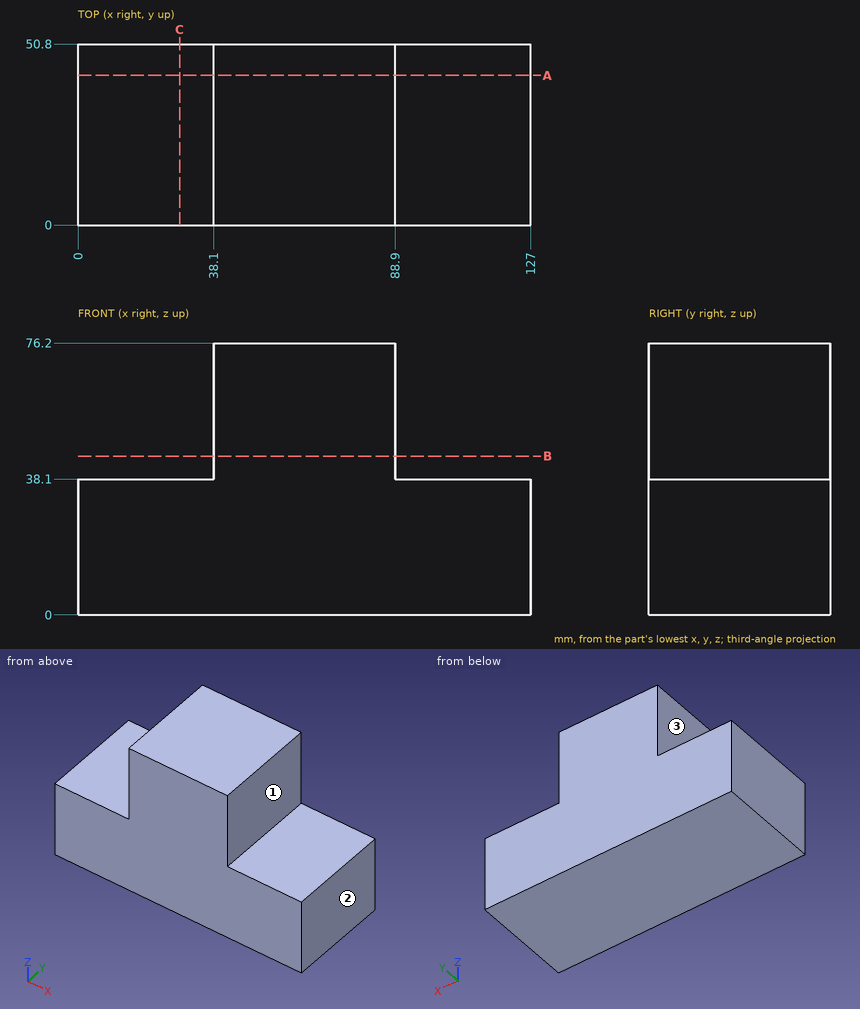
Part print with two shaded views. Sizes in mm from the minimum x, y, z corner. A direction names the side the tool comes from. Coordinates: 2 decimals unless noted, no trailing zeros. Write each loop counter-clockwise with the first axis right and the second up, starting at its lowest first coordinate (ties: lowest second). Pieces come first, ordered by that corner, then holes.
(1) Cut at B-B on z = 44.5. List the corners of the cut face in (x, y).
(2) 3-axis set-ups, long thin cutter, end or side, ignore diameter. For the marked faces 1, 2 and 3: which of +Z, -Z, +X, -X, +Y, -Y reach the whole face in a straight line?
(3) Cut at C-C on x = 28.5. List the corners of the cut face in (y, z).
(4) Drill centre lines: line 1 (X direction, y = 24, z = 68); line 2 (Z direction, x = 101.5, y = 30.5). Where is each one in solid material? Low to high.
(5) Pin check, flat tip, straight feed: pin 1 Ø11.5 at (y, z) = (35.5, 59.5) entering from +X. Stop position of the tip, or through.
(6) Cut at A-A on y = 42. List the corners of the cut face in (x, z), and give its area (3 significant figures).
Working result:
1. outline: (38.1, 0) - (88.9, 0) - (88.9, 50.8) - (38.1, 50.8) - close
2. face 1: +Z, +X, +Y, -Y
2. face 2: +Z, -Z, +X, +Y, -Y
2. face 3: +Z, -X, +Y, -Y
3. outline: (0, 0) - (50.8, 0) - (50.8, 38.1) - (0, 38.1) - close
4. line 1: x = 38.1 to 88.9
4. line 2: z = 0 to 38.1
5. pin 1: stops at x = 88.9
6. outline: (0, 0) - (127, 0) - (127, 38.1) - (88.9, 38.1) - (88.9, 76.2) - (38.1, 76.2) - (38.1, 38.1) - (0, 38.1) - close
6. area: 6,770 mm2
